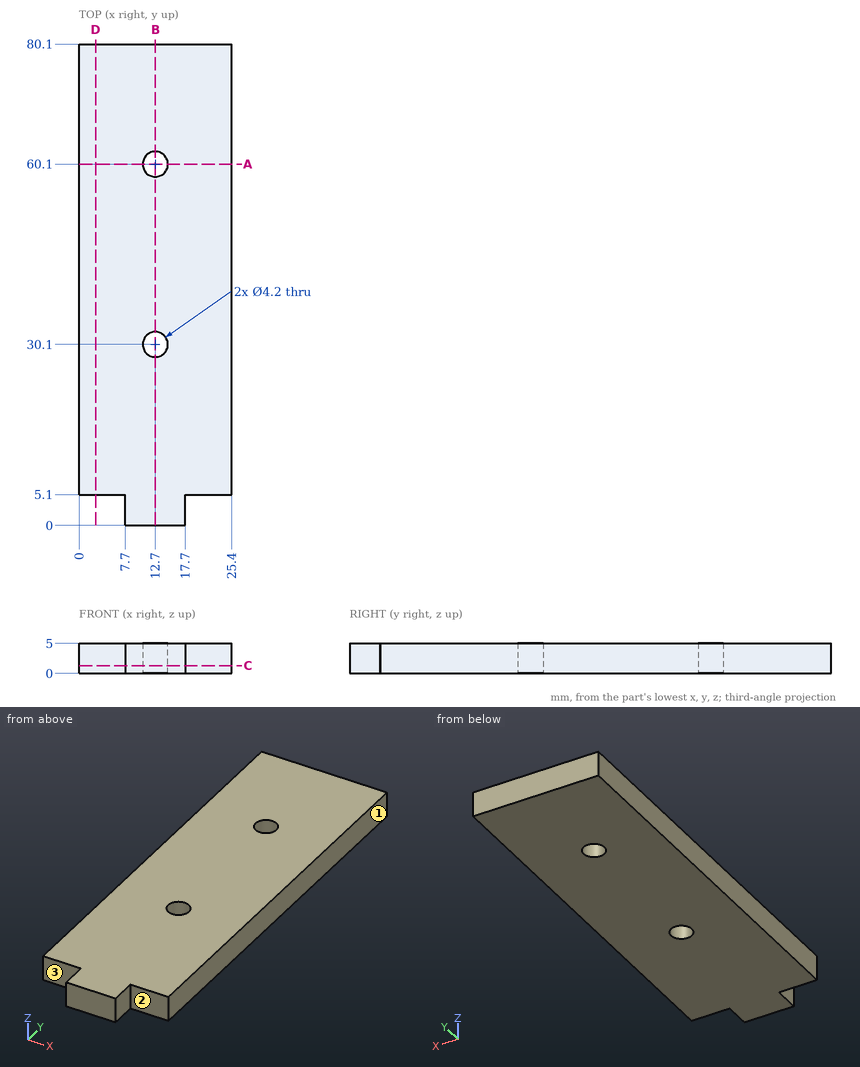
Here's the drawing with two shaded views (mm, measured from the low corner). I have some questions. A direction names the side the tool comes from. Coordinates: 2 decimals unless noted, no trailing zeros. Loops run counter-clockwise (first coordinate to the right, second up) from the corner with the lowest first, then second, coordinate; pieces in that order, holes last. Notation, with made-up numbers: M 21,65.5 L 34,65.5 A11 cw 34,82.5 Z; hole C 65.25,85.25 d8. An arc over 180 degrees is marked long. Put each result on its own line as item: value. Start each with the question number.
(1) Which directions (+Z, -Z, +X, -X, +Y, -Y) give clear straight access to the entire face, cutting with the end or side of a thin tool? Please do the marked faces 1, 2 and 3.
(2) Imagine slicing it at A-A on y = 60.1. List the corners of the cut face in (x, z) for me.
(3) Imagine slicing it at C-C on z = 1.3. List the corners of the cut face in (x, y) for me.
(4) I need wall thicknesses on probe 1 along Y at (x, z) = (12.7, 2.65); probe 2 along Y at (x, z) = (24, 4.3); probe 3 along Y at (x, z) = (13.5, 0.55). Which ranges of each line are inside material? Lowest first, please.
(5) Imagine slicing it at B-B on x = 12.7. List the corners of the cut face in (y, z) for me, and give its area (4 significant figures).
(6) Imagine slicing it at D-D on x = 2.75. List the corners of the cut face in (y, z) for me, and give its area (3 significant figures).
(7) Will these pins go through, and if not, where does the flat tip stop? pin 1 Ø1.5 at (x, z) = (6, 1) entering from -Y; pin 2 Ø3.5 at (x, y) = (12.7, 60.1) entering from -Z; pin 3 Ø1.5 at (y, z) = (1.5, 3.5) entering from -X; pin 4 Ø2.5 at (y, z) = (3.5, 1.5) entering from +X.
Worked answers:
1. face 1: +Z, -Z, +X, +Y, -Y
1. face 2: +Z, -Z, +X, -Y
1. face 3: +Z, -Z, -X, -Y
2. outline: M 0,0 L 10.6,0 L 10.6,5 L 0,5 Z; M 14.8,0 L 25.4,0 L 25.4,5 L 14.8,5 Z
3. outline: M 0,5.1 L 7.7,5.1 L 7.7,0 L 17.7,0 L 17.7,5.1 L 25.4,5.1 L 25.4,80.1 L 0,80.1 Z; hole C 12.7,30.1 d4.2; hole C 12.7,60.1 d4.2
4. probe 1: y = 0 to 28, 32.2 to 58, 62.2 to 80.1
4. probe 2: y = 5.1 to 80.1
4. probe 3: y = 0 to 28.16, 32.04 to 58.16, 62.04 to 80.1
5. outline: M 0,0 L 28,0 L 28,5 L 0,5 Z; M 32.2,0 L 58,0 L 58,5 L 32.2,5 Z; M 62.2,0 L 80.1,0 L 80.1,5 L 62.2,5 Z
5. area: 358.5 mm2
6. outline: M 5.1,0 L 80.1,0 L 80.1,5 L 5.1,5 Z
6. area: 375 mm2
7. pin 1: stops at y = 5.1
7. pin 2: passes through
7. pin 3: stops at x = 7.7
7. pin 4: stops at x = 17.7
